from build123d import *

# Parameters (mm, degrees)
SKETCH1_W           = 142
SKETCH1_H           = 142
BOSS_EXTRUDE1_DEPTH = 60
SKETCH3_W           = 138
SKETCH3_H           = 138
CUT_EXTRUDE1_DEPTH  = 58
SKETCH12_W          = 4
SKETCH12_H          = 50
CUT_EXTRUDE8_DEPTH  = 116.956888541
SKETCH13_R          = 1.5
CUT_EXTRUDE9_DEPTH  = 116.956888541
CUT_EXTRUDE6_REACH  = 171.72
SKETCH9_R           = 5
SKETCH14_R          = 6.363961031
CUT_EXTRUDE10_DEPTH = 169.050587622
CUT_EXTRUDE11_REACH = 171.72
SKETCH16_R          = 13
SKETCH18_R          = 1.5
CUT_EXTRUDE12_DEPTH = 170.720358237
FILLET1_R           = 5
SKETCH19_R          = 1.5
CUT_EXTRUDE13_DEPTH = 170.720358237
SKETCH21_R          = 1.5
CUT_EXTRUDE14_DEPTH = 15


with BuildPart() as part:
    # Sketch1 → Boss-Extrude1 (new body)
    with BuildSketch(Plane(origin=(0, 0, 0), x_dir=(1, 0, 0), z_dir=(0, 1, 0))):
        Rectangle(SKETCH1_W, SKETCH1_H)
    extrude(amount=BOSS_EXTRUDE1_DEPTH)

    # Sketch3 → Cut-Extrude1 (cut)
    with BuildSketch(Plane(origin=(0, 60, 0), x_dir=(1, 0, 0), z_dir=(0, 1, 0))):
        Rectangle(SKETCH3_W, SKETCH3_H)
    extrude(amount=-CUT_EXTRUDE1_DEPTH, mode=Mode.SUBTRACT)

    # Sketch12 → Cut-Extrude8 (cut, through all)
    with BuildSketch(Plane(origin=(0, 2, 0), x_dir=(1, 0, 0), z_dir=(0, 1, 0))):
        with Locations((-65, -42)):
            Rectangle(SKETCH12_W, SKETCH12_H)
        with Locations((-65, 42)):
            Rectangle(SKETCH12_W, SKETCH12_H)
    cut_extrude8 = extrude(amount=-CUT_EXTRUDE8_DEPTH, mode=Mode.SUBTRACT)

    # Mirror2: Cut-Extrude8 across plane
    add(cut_extrude8.mirror(Plane(origin=(0, 0, 0), x_dir=(0, 0, 1), z_dir=(1, 0, 0))), mode=Mode.SUBTRACT)

    # Sketch13 → Cut-Extrude9 (cut, through all)
    with BuildSketch(Plane(origin=(0, 2, 0), x_dir=(1, 0, 0), z_dir=(0, 1, 0))):
        with Locations(Location((-25, -2, 0), (0, 0, 270))):
            Circle(SKETCH13_R)
        with Locations(Location((25, -2, 0), (0, 0, 270))):
            Circle(SKETCH13_R)
        with Locations(Location((25, -52, 0), (0, 0, 270))):
            Circle(SKETCH13_R)
        with Locations(Location((-25, -52, 0), (0, 0, 270))):
            Circle(SKETCH13_R)
        with Locations(Location((-25, 48, 0), (0, 0, 270))):
            Circle(SKETCH13_R)
        with Locations(Location((25, 48, 0), (0, 0, 270))):
            Circle(SKETCH13_R)
    extrude(amount=-CUT_EXTRUDE9_DEPTH, mode=Mode.SUBTRACT)

    # Sketch9 → Cut-Extrude6 (cut, up to next)
    with BuildSketch(Plane(origin=(71, 0, 0), x_dir=(0, 0, -1), z_dir=(1, 0, 0)), mode=Mode.PRIVATE) as cut_extrude6_sk1:
        with Locations((0, 13.5)):
            Circle(SKETCH9_R)
    cut_extrude6_tool1 = extrude(cut_extrude6_sk1.sketch, amount=-CUT_EXTRUDE6_REACH, mode=Mode.PRIVATE) & part.part
    add(cut_extrude6_tool1.solids().sort_by_distance((71, 13.5, 0))[0], mode=Mode.SUBTRACT)

    # Sketch14 → Cut-Extrude10 (cut, through all)
    with BuildSketch(Plane(origin=(0, 0, 69), x_dir=(-1, 0, 0), z_dir=(0, 0, -1))):
        with Locations((21, 44)):
            Circle(SKETCH14_R)
    cut_extrude10 = extrude(amount=-CUT_EXTRUDE10_DEPTH, mode=Mode.SUBTRACT)

    # Mirror3: Cut-Extrude10 across plane
    add(cut_extrude10.mirror(Plane(origin=(0, 0, 0), x_dir=(0, 0, 1), z_dir=(1, 0, 0))), mode=Mode.SUBTRACT)

    # Sketch16 → Cut-Extrude11 (cut, up to next)
    with BuildSketch(Plane.ZY.offset(71), mode=Mode.PRIVATE) as cut_extrude11_sk1:
        with Locations((0, 43)):
            Circle(SKETCH16_R)
    cut_extrude11_tool1 = extrude(cut_extrude11_sk1.sketch, amount=-CUT_EXTRUDE11_REACH, mode=Mode.PRIVATE) & part.part
    add(cut_extrude11_tool1.solids().sort_by_distance((-71, 43, 0))[0], mode=Mode.SUBTRACT)

    # Sketch18 → Cut-Extrude12 (cut, through all)
    with BuildSketch(Plane.ZY.offset(71)):
        with Locations((-46, 15)):
            Circle(SKETCH18_R)
        with Locations((46, 15)):
            Circle(SKETCH18_R)
    extrude(amount=-CUT_EXTRUDE12_DEPTH, mode=Mode.SUBTRACT)

    # Fillet1
    fillet1_edges = [part.edges().sort_by_distance(p)[0] for p in [
        (-69, 31, 69),
        (-69, 31, -69),
        (69, 31, -69),
        (69, 31, 69),
        (71, 30, 71),
        (-71, 30, 71),
        (-71, 30, -71),
        (71, 30, -71),
    ]]
    fillet(fillet1_edges, radius=FILLET1_R)

    # Sketch19 → Cut-Extrude13 (cut, through all)
    with BuildSketch(Plane.ZY.offset(71)):
        with Locations((-40, 57)):
            Circle(SKETCH19_R)
        with Locations((40, 57)):
            Circle(SKETCH19_R)
    extrude(amount=-CUT_EXTRUDE13_DEPTH, mode=Mode.SUBTRACT)

    # Sketch21 → Cut-Extrude14 (cut)
    with BuildSketch(Plane.XY.offset(-71)):
        with Locations(Location((-12, 24.5, 0), (0, 0, 180))):
            Circle(SKETCH21_R)
        with Locations(Location((12, 24.5, 0), (0, 0, 180))):
            Circle(SKETCH21_R)
    extrude(amount=CUT_EXTRUDE14_DEPTH, mode=Mode.SUBTRACT)


solid = part.part
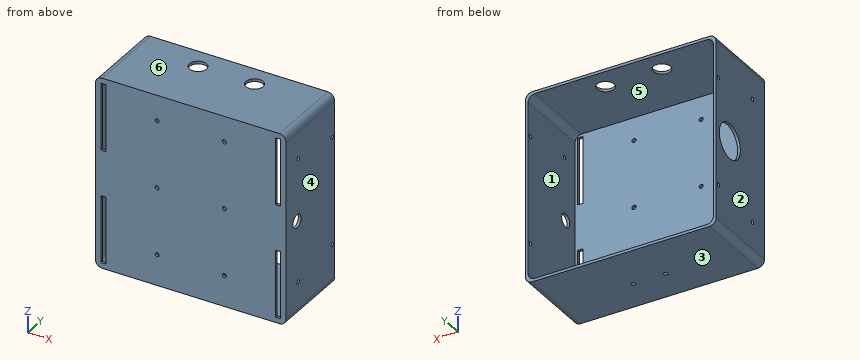
Here's how the part is built. I have some questions about the finished solid (model axes, mm). Face numbers are marked on the shaded views. A direction names the side the tool comes from. Coordinates: 2 decimals unless noted, no trailing zeros. Order: outer loops, then holes, each group sorted by start corner. A loop starts at its lowest first (then second) coordinate and runs counter-clockwise, first axis right, second up. Notation, with made-up numbers: (81.5, 16) -> (91.5, 16) arc R11 ccw to (91.5, 24) -> close; hole circle Ø1 at (75.25, -28). An arc over 180 degrees is marked (long way). Answer in a Markdown table with one row per item.
(1) Please list where these lines run through material, in increasing order: probe 1 along Z at (x, y) = (47.5, 27.5); probe 2 along Y at (x, z) = (-70, 0).
Answer key:
| item | result |
|---|---|
| probe 1 | -71 to -69, 69 to 71 |
| probe 2 | 0 to 30, 56 to 60 |
(2) I want a section at C-C on z = 22. List the corners of the cut face in (x, y) for me, then the cut area to 3 significant figures.
Answer key:
| item | result |
|---|---|
| outline | (-71, 0) -> (-67, 0) -> (-67, 2) -> (-69, 2) -> (-69, 60) -> (-71, 60) -> close; (-63, 0) -> (63, 0) -> (63, 2) -> (-63, 2) -> close; (67, 0) -> (71, 0) -> (71, 60) -> (69, 60) -> (69, 2) -> (67, 2) -> close |
| area | 500 mm^2 |
(3) Will this pin go through, and if not, where does the flat tip stop? pin 1 Ø4 at (x, z) = (25, 52) entering from +Y.
Answer key:
| item | result |
|---|---|
| pin 1 | y = 2 |
(4) I want a section at B-B on x = -21. List the corners of the cut face in (y, z) for me, then the cut area to 3 significant figures.
Answer key:
| item | result |
|---|---|
| outline | (0, -71) -> (60, -71) -> (60, -69) -> (2, -69) -> (2, 69) -> (37.64, 69) -> (37.64, 71) -> (0, 71) -> close; (50.36, 69) -> (60, 69) -> (60, 71) -> (50.36, 71) -> close |
| area | 491 mm^2 |
(5) I want a section at A-A on y = 6. List the corners of the cut face in (x, z) for me.
Answer key:
| item | result |
|---|---|
| outline | (-71, -66) arc R5 ccw to (-66, -71) -> (66, -71) arc R5 ccw to (71, -66) -> (71, 66) arc R5 ccw to (66, 71) -> (-66, 71) arc R5 ccw to (-71, 66) -> close; hole (-69, -64) arc R5 ccw to (-64, -69) -> (64, -69) arc R5 ccw to (69, -64) -> (69, 64) arc R5 ccw to (64, 69) -> (-64, 69) arc R5 ccw to (-69, 64) -> close |
(6) I want a section at D-D on y = 40. List the corners of the cut face in (x, z) for me.
Answer key:
| item | result |
|---|---|
| outline | (-71, -66) arc R5 ccw to (-66, -71) -> (66, -71) arc R5 ccw to (71, -66) -> (71, 66) arc R5 ccw to (66, 71) -> (25.95, 71) -> (25.95, 69) -> (64, 69) arc R5 cw to (69, 64) -> (69, -64) arc R5 cw to (64, -69) -> (-64, -69) arc R5 cw to (-69, -64) -> (-69, -12.65) -> (-71, -12.65) -> close; (-71, 12.65) -> (-69, 12.65) -> (-69, 64) arc R5 cw to (-64, 69) -> (-25.95, 69) -> (-25.95, 71) -> (-66, 71) arc R5 ccw to (-71, 66) -> close; (-16.05, 69) -> (16.05, 69) -> (16.05, 71) -> (-16.05, 71) -> close |
(7) Thinking about a two-plate mould opening in X: for the marked faces 1, 2, 3 and 4, which applies, +X half, -X half, draft (parallel to the pull), parting line (faces both ways), or undercut?
Answer key:
| item | result |
|---|---|
| face 1 | undercut |
| face 2 | -X half |
| face 3 | draft |
| face 4 | +X half |
(8) On a 3-axis mill with a long thin cutter (end or side, diameter ignored), from which of +Z, -Z, +X, -X, +Y, -Y can I reach the whole of each face in a straight line? I mean the marked faces 5 and 6. Say none if no direction works.
Answer key:
| item | result |
|---|---|
| face 5 | +Y |
| face 6 | +Z, +X, -X, +Y, -Y |
